```python
from build123d import *

# Parameters (mm, degrees)
P_IDAT_VYSUNUT_M1_DEPTH  = 19
SKICA2_W                 = 4
SKICA2_H                 = 4
ODEBRAT_VYSUNUT_M1_DEPTH = 15
SKICA3_W                 = 32
SKICA3_H                 = 15
ODEBRAT_VYSUNUT_M2_DEPTH = 1
SKICA4_W                 = 4
SKICA4_H                 = 4
ODEBRAT_VYSUNUT_M3_DEPTH = 50
SKICA5_W                 = 4
SKICA5_H                 = 3
P_IDAT_VYSUNUT_M2_DEPTH  = 5
SKICA6_R                 = 2
ODEBRAT_VYSUNUT_M4_DEPTH = 5
SKICA8_W                 = 4
SKICA8_H                 = 3
ODEBRAT_VYSUNUT_M6_DEPTH = 5
SKICA9_W                 = 4
SKICA9_H                 = 3
P_IDAT_VYSUNUT_M3_DEPTH  = 5


with BuildPart() as part:
    # Skica1 → Přidat vysunutím1 (new body)
    with BuildSketch(Plane.XY):
        Polygon((0, 0), (0, 7), (4, 7), (4, 3), (36, 3), (36, 0), align=None)
    extrude(amount=P_IDAT_VYSUNUT_M1_DEPTH)

    # Skica2 → Odebrat vysunutím1 (cut)
    with BuildSketch(Plane.XY.offset(19)):
        with Locations((2, 5)):
            Rectangle(SKICA2_W, SKICA2_H)
    extrude(amount=-ODEBRAT_VYSUNUT_M1_DEPTH, mode=Mode.SUBTRACT)

    # Skica3 → Odebrat vysunutím2 (cut)
    with BuildSketch(Plane.XZ):
        with Locations((18, 9.5)):
            Rectangle(SKICA3_W, SKICA3_H)
    extrude(amount=-ODEBRAT_VYSUNUT_M2_DEPTH, mode=Mode.SUBTRACT)

    # Skica4 → Odebrat vysunutím3 (cut)
    with BuildSketch(Plane.ZY):
        with Locations((2, 5)):
            Rectangle(SKICA4_W, SKICA4_H)
    extrude(amount=-ODEBRAT_VYSUNUT_M3_DEPTH, mode=Mode.SUBTRACT)

    # Skica5 → Přidat vysunutím2 (add)
    with BuildSketch(Plane.ZY):
        with Locations((2, 1.5)):
            Rectangle(SKICA5_W, SKICA5_H)
    extrude(amount=P_IDAT_VYSUNUT_M2_DEPTH)

    # Skica6 → Odebrat vysunutím4 (cut)
    with BuildSketch(Plane.XZ.offset(-1)):
        with Locations((27, 9.5)):
            Circle(SKICA6_R)
    extrude(amount=-ODEBRAT_VYSUNUT_M4_DEPTH, mode=Mode.SUBTRACT)

    # Skica8 → Odebrat vysunutím6 (cut)
    with BuildSketch(Plane.ZY.offset(5)):
        with Locations((2, 1.5)):
            Rectangle(SKICA8_W, SKICA8_H)
    extrude(amount=-ODEBRAT_VYSUNUT_M6_DEPTH, mode=Mode.SUBTRACT)

    # Skica9 → Přidat vysunutím3 (add)
    with BuildSketch(Plane.ZY):
        with Locations((17, 1.5)):
            Rectangle(SKICA9_W, SKICA9_H)
    extrude(amount=P_IDAT_VYSUNUT_M3_DEPTH)


solid = part.part
```
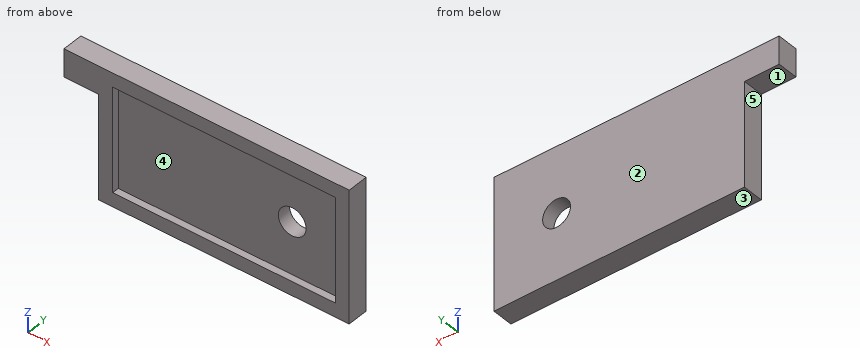
Geometry check sheet. Reference: the model listing, model coordinates, mm. Face numbers are marked on the shaded views. A direction names the side the tool comes from. Round coordinates to 2 decimals unless told otherwise and drop trailing zeros. Order: outer loops, then holes, each group sorted by start corner. A loop starts at its lowest first (then second) coordinate and runs counter-clockwise, first axis right, second up. Notation, with made-up numbers: (-17.5, 9.5) - (-0.5, 9.5) arc R31 cw to (-0.5, 34.5) - close; hole circle Ø8 at (26, -22.5). An arc over 180 degrees is marked (long way). Use a Markdown table: item, result. Add a question column.
1) Gauge pin test, flat ends, axial feed: P1, Ø3, axis at x = 26.5, z = 6, coming from the -Y side; P2, Ø0.9, axis at x = -2, y = 1, coming from the -Z side; P3, Ø0.8, axis at y = 0.5, z = 7, coming from the -X side. Record the tip position at first contact, or that the pin passes through.
2) Section check A-A (z = 9.5). Record the cut outline in (x, y), then the cut area to 3 significant figures.
3) Section check B-B (x = 27). Record the cut outline in (y, z), then the cut area to 3 significant figures.
4) Set-up check for the marked faces 1 and 2: record each of +Z, -Z, +X, -X, +Y, -Y from which the full face is reachable in a straight line by a thin tool's end or side.
5) Section check C-C (y = 2.35). Record the cut outline in (x, z).
6) Thickness scan on line 1 along Z through (x, y) = (27, 2.15); line 2 along X through (y, z) = (0.4, 14.75); line 3 along Z through (x, y) = (9.5, 0.9). Record the ranges inside material, lowest first.
7) Mould release check, pull along X, two halves, no side actions. Record for the marked faces 3, 4 and 5: released by +X, released by -X, zero draft, split by the parting line, or undercut.
8) Section check D-D (z = 6). Record the cut outline in (x, y).
Established:
| question | item | result |
|---|---|---|
| 1 | P1 | y = 1 |
| 1 | P2 | z = 15 |
| 1 | P3 | x = 0 |
| 2 | outline | (0, 0) - (2, 0) - (2, 1) - (25, 1) - (25, 3) - (0, 3) - close; (29, 1) - (34, 1) - (34, 0) - (36, 0) - (36, 3) - (29, 3) - close |
| 2 | area | 68.0 mm2 |
| 3 | outline | (0, 0) - (3, 0) - (3, 7.5) - (1, 7.5) - (1, 2) - (0, 2) - close; (0, 17) - (1, 17) - (1, 11.5) - (3, 11.5) - (3, 19) - (0, 19) - close |
| 3 | area | 34.0 mm2 |
| 4 | face 1 | -Z, -X, +Y, -Y |
| 4 | face 2 | +Z, -Z, +X, -X, +Y |
| 5 | outline | (-5, 15) - (0, 15) - (0, 0) - (36, 0) - (36, 19) - (-5, 19) - close; hole circle Ø4 at (27, 9.5) |
| 6 | line 1 | 0 to 7.5, 11.5 to 19 |
| 6 | line 2 | 0 to 2, 34 to 36 |
| 6 | line 3 | 0 to 2, 17 to 19 |
| 7 | face 3 | zero draft |
| 7 | face 4 | undercut |
| 7 | face 5 | released by -X |
| 8 | outline | (0, 0) - (2, 0) - (2, 1) - (34, 1) - (34, 0) - (36, 0) - (36, 3) - (0, 3) - close |
